Source: CAD feature listing. Evaluate the final solid. Frame: model axes, mm. A direction names the side the tool comes from. Coordinates: 2 decimals unless noted, no trailing zeros. Order: outer loops, then holes, each group sorted by start corner. A loop starts at its lowest first (then second) coordinate and runs counter-clockwise, first axis right, second up. Notation, with made-up numbers: (83.5, 82.5) -> (133.5, 82.5) arc R9 ccw to (133.5, 91.5) -> close; hole circle Ø10 at (-36, -14.5). An arc over 180 degrees is marked (long way). Write each question's results on one line, items separated by ' | '. Start each with the question number.
from build123d import *

# Parameters (mm, degrees)
SKETCH1_W             = 11.94
SKETCH1_H             = 11.94
BOSS_EXTRUDE1_DEPTH   = 1.14
CUT_EXTRUDE2_DEPTH    = 12.94
LPATTERN1_COUNT       = 2
LPATTERN1_PITCH       = 2
LPATTERN1_COL_COUNT   = 2
LPATTERN1_COL_PITCH   = 2
SKETCH7_W             = 1.14
SKETCH7_H             = 11.94
BOSS_EXTRUDE2_DEPTH   = 11.51
BOSS_EXTRUDE3_DEPTH   = 1.52
LPATTERN3_COUNT       = 3
LPATTERN3_PITCH       = 5.21
MIRROR1_COPY_1_DEPTH  = 1.52
MIRROR1_COPY_2_DEPTH  = 1.52
FILLET2_R             = 1.14
M5X0_8_TAPPED_HOLE2_D = 4.2


with BuildPart() as part:
    # Sketch1 → Boss-Extrude1 (new body)
    with BuildSketch(Plane(origin=(0, 0, 0), x_dir=(1, 0, 0), z_dir=(0, 1, 0))):
        Rectangle(SKETCH1_W, SKETCH1_H)
    extrude(amount=BOSS_EXTRUDE1_DEPTH)

    # Sketch4 → Cut-Extrude2 (cut, through all)
    with BuildSketch(Plane.XY.offset(5.97)):
        Polygon((0.2, 1.14), (0.5, 0.84), (0.8, 1.14), align=None)
        Polygon((-0.5, 0.84), (-0.2, 1.14), (-0.8, 1.14), align=None)
    cut_extrude2 = extrude(amount=-CUT_EXTRUDE2_DEPTH, mode=Mode.SUBTRACT)

    # LPattern1: Cut-Extrude2 ×2
    with Locations(*[(i * LPATTERN1_PITCH, 0, 0) for i in range(1, LPATTERN1_COUNT)]):
        add(cut_extrude2, mode=Mode.SUBTRACT)

    # LPattern1 col: Cut-Extrude2 ×2
    with Locations(*[(-i * LPATTERN1_COL_PITCH, 0, 0) for i in range(1, LPATTERN1_COL_COUNT)]):
        add(cut_extrude2, mode=Mode.SUBTRACT)

    # Sketch7 → Boss-Extrude2 (add)
    with BuildSketch(Plane.XZ):
        with Locations((-5.4, 0)):
            Rectangle(SKETCH7_W, SKETCH7_H)
        with Locations((5.4, 0)):
            Rectangle(SKETCH7_W, SKETCH7_H)
    extrude(amount=BOSS_EXTRUDE2_DEPTH)

    # Sketch6 → Boss-Extrude3 (add)
    with BuildSketch(Plane.XY.offset(5.97)):
        with BuildLine():
            Line((-4.83, -11.51), (-4.83, -11.86806677))
            ThreePointArc((-4.83, -11.86806677), (-5.321138867, -13.595029247), (-4.418877615, -15.14729901))
            Line((-4.418877615, -15.14729901), (-5.101941963, -16.06))
            ThreePointArc((-5.101941963, -16.06), (-6.41810343, -13.95329498), (-5.97, -11.51))
            Line((-5.97, -11.51), (-4.83, -11.51))
        make_face()
    boss_extrude3 = extrude(amount=-BOSS_EXTRUDE3_DEPTH)

    # LPattern3: Boss-Extrude3 ×3
    with Locations(*[(0, 0, -i * LPATTERN3_PITCH) for i in range(1, LPATTERN3_COUNT)]):
        add(boss_extrude3)

    # Mirror1: Boss-Extrude3 across plane
    add(boss_extrude3.mirror(Plane(origin=(0, 0, 0), x_dir=(0, 0, 1), z_dir=(1, 0, 0))))

    # Mirror1 copy 1 sketch → Mirror1 copy 1 (add)
    with BuildSketch(Plane(origin=(0, 0, 0.76), x_dir=(-1, 0, 0), z_dir=(0, 0, 1))):
        with BuildLine():
            Line((-4.83, 11.51), (-4.83, 11.86806677))
            ThreePointArc((-4.83, 11.86806677), (-5.321138867, 13.595029247), (-4.418877615, 15.14729901))
            Line((-4.418877615, 15.14729901), (-5.101941963, 16.06))
            ThreePointArc((-5.101941963, 16.06), (-6.41810343, 13.95329498), (-5.97, 11.51))
            Line((-5.97, 11.51), (-4.83, 11.51))
        make_face()
    extrude(amount=-MIRROR1_COPY_1_DEPTH)

    # Mirror1 copy 2 sketch → Mirror1 copy 2 (add)
    with BuildSketch(Plane(origin=(0, 0, -4.45), x_dir=(-1, 0, 0), z_dir=(0, 0, 1))):
        with BuildLine():
            Line((-4.83, 11.51), (-4.83, 11.86806677))
            ThreePointArc((-4.83, 11.86806677), (-5.321138867, 13.595029247), (-4.418877615, 15.14729901))
            Line((-4.418877615, 15.14729901), (-5.101941963, 16.06))
            ThreePointArc((-5.101941963, 16.06), (-6.41810343, 13.95329498), (-5.97, 11.51))
            Line((-5.97, 11.51), (-4.83, 11.51))
        make_face()
    extrude(amount=-MIRROR1_COPY_2_DEPTH)

    # Fillet2
    fillet2_edges = [part.edges().sort_by_distance(p)[0] for p in [
        (5.97, 1.14, 0),
        (-5.97, 1.14, 0),
    ]]
    fillet(fillet2_edges, radius=FILLET2_R)

    # M5x0.8 Tapped Hole2 (through all)
    with Locations(Plane.XZ):
        with Locations((0, 0)):
            Hole(M5X0_8_TAPPED_HOLE2_D / 2)


solid = part.part
(1) Section D-D on y = -13. Return the cut outline in (x, z) (3 decimals), then the cut area to 3 significant figures.
(2) Section A-A on x = 0. Return the cut outline in (y, z), then the cut area to 3 significant figures.
(3) Draft query along Y for faces 1 (the flat face through (6, -14, -4.45)), 2 (the cylindrical face through (5.324, -13.569, 5.221)), 3 (the flat face through (-4.76, -15.6, 5.22)), 4 (the cylindrical face through (-5.324, -13.569, 5.221)). Return one class per face: released by +Y, released by -Y, zero draft, split by the parting line, or undercut.
(4) Section C-C on y = -10. Return the cut outline in (x, z), then the cut area to 3 significant figures.
(5) Line query: L1, parallel to X at y = -3.5, z = -3.5; L2, parallel to Z at x = 0, y = 0.25; L3, parallel to Y at x = 3, z = -4.5. Output: solid intervals per line, ascending.
(6) Section B-B on z = 0. Return the cut outline in (x, y), then the cut area to 3 significant figures.
(7) Reachability of faces 5 (the flat face through (5, -11.51, 3)), 6 (the flat face through (4.76, -15.6, 0.01)), 7 (the cylindrical face through (5.324, -13.569, 0.011)) from +Z, -Z, +X, -X, +Y, -Y: full face, straight path, thin tool, end or side. Return the list, or none.
(8) First-contact query: P1, Ø6, axis at y = -7, z = -2.5, coming from the +X side; P2, Ø5.5, axis at x = 0, z = 0, coming from the -Y side; P3, Ø0.6, axis at x = -5, z = -2.5, coming from the -Y side. Flat tips, straight axial feed; report the tip coordinate or a pass-through.
Results list:
1) outline: (-6.465, -5.97) -> (-5.318, -5.97) -> (-5.318, -4.45) -> (-6.465, -4.45) -> close; (-6.465, -0.76) -> (-5.318, -0.76) -> (-5.318, 0.76) -> (-6.465, 0.76) -> close; (-6.465, 4.45) -> (-5.318, 4.45) -> (-5.318, 5.97) -> (-6.465, 5.97) -> close; (5.318, -5.97) -> (6.465, -5.97) -> (6.465, -4.45) -> (5.318, -4.45) -> close; (5.318, -0.76) -> (6.465, -0.76) -> (6.465, 0.76) -> (5.318, 0.76) -> close; (5.318, 4.45) -> (6.465, 4.45) -> (6.465, 5.97) -> (5.318, 5.97) -> close | area: 10.5 mm²
2) outline: (0, -5.97) -> (1.14, -5.97) -> (1.14, -2.1) -> (0, -2.1) -> close; (0, 2.1) -> (1.14, 2.1) -> (1.14, 5.97) -> (0, 5.97) -> close | area: 8.82 mm²
3) face 1: zero draft | face 2: undercut | face 3: released by -Y | face 4: undercut
4) outline: (-5.97, -5.97) -> (-4.83, -5.97) -> (-4.83, 5.97) -> (-5.97, 5.97) -> close; (4.83, -5.97) -> (5.97, -5.97) -> (5.97, 5.97) -> (4.83, 5.97) -> close | area: 27.2 mm²
5) L1: x = -5.97 to -4.83, 4.83 to 5.97 | L2: z = -5.97 to -2.1, 2.1 to 5.97 | L3: y = 0 to 1.14
6) outline: (-5.97, -11.51) arc R3.44 ccw to (-5.1, -16.06) -> (-4.42, -15.15) arc R2.3 cw to (-4.83, -11.87) -> (-4.83, 0) -> (-2.1, 0) -> (-2.1, 1.14) -> (-2.2, 1.14) -> (-2.5, 0.84) -> (-2.8, 1.14) -> (-4.83, 1.14) arc R1.14 ccw to (-5.97, 0) -> close; (2.1, 0) -> (4.83, 0) -> (4.83, -11.87) arc R2.3 cw to (4.42, -15.15) -> (5.1, -16.06) arc R3.44 ccw to (5.97, -11.51) -> (5.97, 0) arc R1.14 ccw to (4.83, 1.14) -> (2.8, 1.14) -> (2.5, 0.84) -> (2.2, 1.14) -> (2.1, 1.14) -> close | area: 44.7 mm²
7) face 5: +X, -X, -Y | face 6: +Z, -Z, -Y | face 7: +Z, -Z
8) P1: stops at x = 5.97 | P2: stops at y = 0 | P3: stops at y = -11.51
